Solid Edge part; units mm, degrees
sketch "Sketch1" plane through (10.8674, 0, 10.8674) normal (0, -1, 0) x (1, 0, 0)
  line L0 (-31.8306, -10.8674) -> (-31.8306, 9.6326)
  line L1 (-31.8306, 9.6326) -> (-21.8306, 9.6326)
  line L2 (-21.8306, 9.6326) -> (-17.099, -3.3674)
  line L3 (-17.099, -3.3674) -> (-16.099, -3.3674)
  line L4 (-16.099, -3.3674) -> (-11.3674, 9.6326)
  line L5 (-11.3674, 9.6326) -> (-10.3674, 9.6326)
  line L6 (-10.3674, 9.6326) -> (-5.6358, -3.3674)
  line L7 (-5.6358, -3.3674) -> (-4.6358, -3.3674)
  line L8 (-4.6358, -3.3674) -> (0.0958, 9.6326)
  line L9 (0.0958, 9.6326) -> (1.0958, 9.6326)
  line L10 (1.0958, 9.6326) -> (6.7374, -5.8674)
  line L11 (6.7374, -5.8674) -> (12.6194, -5.8674)
  line L12 (12.6194, -5.8674) -> (12.6194, -10.8674)
  dimension "D1" = 31.8306
  dimension "D2" = 31.8306
  dimension "D3" = 11.3674
  dimension "D4" = 17.099
revolve "RevolvedProtrusion1" add sketch "Sketch1" angle 360 about axis through (-17.7633, 0, 0) along (1, 0, 0)
shell "Thinwall1" thickness 0.5 removed faces 1 at (-20.9632, 13.2567, 14.0767)
sketch "Sketch2" plane through (23.4868, 0, 0) normal (1, 0, 0) x (0, -1, 0)
  circle A0 centre (0, 0) radius 4
extrude "Cutout1" cut sketch "Sketch2" against normal through all
properties material "Steel"
The model under review builds one solid part; all positions refer to its coordinate system, in mm. A direction names the side the tool comes from. Coordinates: 2 decimals unless noted, no trailing zeros. Loops run counter-clockwise (first coordinate to the right, second up) from the corner with the lowest first, then second, coordinate; pieces in that order, holes last. Notation, with made-up numbers: (21.25, 55) -> (64.25, 55) arc R23 cw to (64.25, 73) -> close; hole circle Ø2 at (-25, 89). An arc over 180 degrees is marked (long way). Answer as CSV lines item,"result".
Item 1: Draft analysis for pull direction Z (two halves, no side actions). For faces 1 (the flat face through (-20.963, 9, 18.1)), 2 (the cylindrical face through (20.16, -4.46, -0.59)), 3 (the conical face through (-4.936, -5.618, -6.127)), state which applies: +Z half, -Z half, draft (parallel to the pull), parting line (faces both ways), or undercut.
Results below:
face 1,"draft"
face 2,"undercut"
face 3,"parting line"
Item 2: Machinability: for faces 4 (the cylindrical face through (0.007, 20.013, -4.444)), 5 (the cylindrical face through (20.59, 4.88, -1.08)), 6 (the conical face through (4.586, -7.627, -1.694)), 7 (the flat face through (22.987, 3, -3)), which of the approach directions +Z, -Z, +X, -X, +Y, -Y give a long, thin tool a straight path to every point of the face, cutting with its end or side? Answer none if there is none.
Results below:
face 4,"+X, -X"
face 5,"+X"
face 6,"none"
face 7,"-X"
Item 3: For L1, parallel to X at y = 8, z = -14; L2, parallel to Y at x = 23.35, z = 0; L3, parallel to Y at x = -15, z = 0, list the stretches that pass through material, from the lowest coordinate up.
Results below:
L1,"x = -9.9 to -9.37, -2.09 to -1.56, 1.56 to 2.09, 9.37 to 9.9, 13.02 to 13.56"
L2,"y = -5 to -4, 4 to 5"
L3,"y = -20.5 to -20, 20 to 20.5"
Item 4: Insertion check: pin 1 (5 mm diameter, centred on y = -6, z = -11, fed in from +X); pin 2 (1.5 mm diameter, centred on y = -13.5, z = -0.5, fed in from -X); pin 3 (8 mm diameter, centred on y = 5, z = 15, fed in from -X). Each pin has a flat end and moves straight along its axis. Give the tip position at first contact, or say it passes through.
Results below:
pin 1,"stops at x = 15.77"
pin 2,"stops at x = -9.22"
pin 3,"stops at x = -11.24"
Item 5: Take a section at A-A, the plane y = -16. Count the separate pieces of the cut face and the enclosed holes in it, and give its area (3 significant figures).
Results below:
separate pieces,"3"
enclosed holes,"2"
area,"84.2 mm2"
Item 6: Take a section at B-B, the plane x = -14. State the section outline as (y, z) points, and give its area (3 significant figures).
Results below:
outline,"circle Ø41 at (0, 0); hole circle Ø40 at (0, 0)"
area,"63.6 mm2"
